```python
from build123d import *

# Parameters (mm, degrees)
SKETCH074_W     = 13
SKETCH074_H     = 5
PAD037_DEPTH    = 1
SKETCH070_R     = 1.5
PAD038_DEPTH    = 2
FILLET010_R     = 1.5
SKETCH073_W     = 0.5
SKETCH073_H     = 4
SKETCH073_W_2   = 4
SKETCH073_H_2   = 0.5
POCKET025_DEPTH = 1.5


with BuildPart() as part:
    # Sketch074 (on Face1 of CopyPocket001) → Pad037 (new body)
    with BuildSketch(Plane.XY.offset(8.15)):
        with Locations((7, -24)):
            Rectangle(SKETCH074_W, SKETCH074_H)
    extrude(amount=PAD037_DEPTH)

    # Sketch070 (on Face6 of Pad037) → Pad038 (join)
    with BuildSketch(Plane.XY.offset(9.15)):
        with Locations((3, -24)):
            Circle(SKETCH070_R)
        with Locations((11, -24)):
            Circle(SKETCH070_R)
    extrude(amount=PAD038_DEPTH)

    # Fillet010
    fillet010_edges = [part.edges().sort_by_distance(p)[0] for p in [
        (9.5, -24, 11.15),
        (1.5, -24, 11.15),
    ]]
    fillet(fillet010_edges, radius=FILLET010_R)

    # Sketch073 (on Face12 of Fillet010) → Pocket025 (cut)
    with BuildSketch(Plane.XY.offset(11.15)):
        with Locations((3, -24)):
            Rectangle(SKETCH073_W, SKETCH073_H)
        with Locations((11, -24)):
            Rectangle(SKETCH073_W_2, SKETCH073_H_2)
    extrude(amount=-POCKET025_DEPTH, mode=Mode.SUBTRACT)


solid = part.part
```
The model under review builds one solid part; all positions refer to its coordinate system, in mm. A direction names the side the tool comes from. Give positions to 0.01 mm unless a question says otherwise; leave off trailing zeros. Order: outer loops, then holes, each group sorted by start corner. A loop starts at its lowest first (then second) coordinate and runs counter-clockwise, first axis right, second up. Notation, with made-up numbers: (51.5, 8) - (56.5, 8) arc R15 cw to (56.5, 25) - close; hole circle Ø11 at (77.25, -6.75). An arc over 180 degrees is marked (long way). Use CSV: the item, a comma, the result in double quotes. Start each with the question number.
Q1. We need section D-D, the plane z = 9.4. Write out the cut boundary in (x, y), and give its area (3 significant figures).
Q2. We need section A-A, the plane z = 10.3. Write out the cut boundary in (x, y), and give its area (3 significant figures).
Q3. Tool access review of faces 1 (the flat face through (7, -24, 9.15)), 2 (the flat face through (11, -24.25, 10)), 3 (the flat face through (3.25, -24, 10)): name each direction out of +Z, -Z, +X, -X, +Y, -Y from which nothing blocks a thin tool from reaching the whole face with its end or side.
Q4. To check wall thickness, follow line 1 along X through (y, z) = (-23.65, 10.15); line 2 along X through (y, z) = (-24.45, 10.6); line 3 along Y through (x, z) = (3, 9.5). State the ranges of each line that lie inside material, in increasing order. Write a range as [from, to].
Q5. The part is to be moulded in two halves that separate along Y. For faces 4 (the flat face through (7, -26.5, 9)), 5 (the flat face through (0.5, -24, 9)), 6 (the flat face through (11, -23.75, 10)), 7 (the cylindrical face through (2.805, -22.513, 9.396)), say which applies: +Y half, -Y half, draft (parallel to the pull), parting line (faces both ways), or undercut.
Q6. We need section C-C, the plane y = -24. Write out the cut boundary in (x, z), and give its area (3 significant figures).
Q7. Clearance check with flat-ended pins moving along their axes: pin 1 Ø1.6 at (y, z) = (-24, 10) entering from -X; pin 2 Ø1.5 at (y, z) = (-22, 10) entering from -X; pin 3 Ø0.6 at (x, y) = (11, -24) entering from +Z; pin 4 Ø1.2 at (x, z) = (10.5, 10.5) entering from -Y. State where each tip first meets the part, or that it passes through.
Q8. We need section B-B, the plane x = 3. Write out the cut boundary in (y, z), and give its area (3 significant figures).
Outcome:
1,outline,"circle Ø3 at (3, -24); circle Ø3 at (11, -24)"
1,area,"14.1 mm^2"
2,outline,"(2.75, -25.33) - (2.75, -22.67) arc R1.35 ccw to start; (3.25, -25.33) arc R1.35 ccw to (3.25, -22.67) - close; (9.67, -24.25) arc R1.35 ccw to (12.33, -24.25) - close; (9.67, -23.75) - (12.33, -23.75) arc R1.35 ccw to start"
2,area,"8.79 mm^2"
3,face 1,"+Z"
3,face 2,"+Z, +X"
3,face 3,"+Z, +Y, -Y"
4,line 1,"x = [1.63, 2.75], [3.25, 4.37], [9.63, 12.37]"
4,line 2,"x = [1.93, 2.75], [3.25, 4.07], [9.93, 12.07]"
4,line 3,"y = [-25.5, -22.5]"
5,face 4,"-Y half"
5,face 5,"draft"
5,face 6,"undercut"
5,face 7,"parting line"
6,outline,"(0.5, 8.15) - (13.5, 8.15) - (13.5, 9.15) - (12.5, 9.15) - (12.5, 9.65) - (9.5, 9.65) - (9.5, 9.15) - (4.5, 9.15) - (4.5, 9.65) arc R1.5 ccw to (3.25, 11.13) - (3.25, 9.65) - (2.75, 9.65) - (2.75, 11.13) arc R1.5 ccw to (1.5, 9.65) - (1.5, 9.15) - (0.5, 9.15) - close"
6,area,"18.8 mm^2"
7,pin 1,"stops at x = 1.5"
7,pin 2,"stops at x = 2.22"
7,pin 3,"stops at z = 11.13"
7,pin 4,"stops at y = -25.45"
8,outline,"(-26.5, 8.15) - (-21.5, 8.15) - (-21.5, 9.15) - (-22.5, 9.15) - (-22.5, 9.65) - (-25.5, 9.65) - (-25.5, 9.15) - (-26.5, 9.15) - close"
8,area,"6.50 mm^2"
